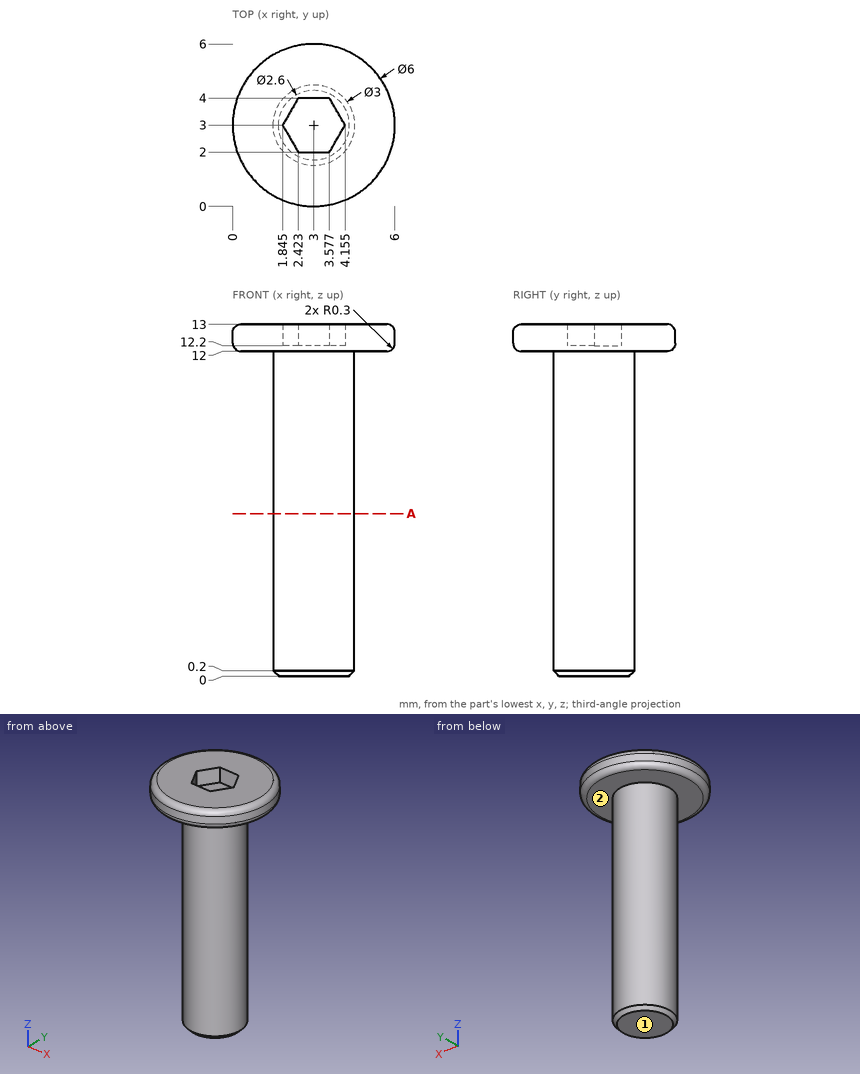
Study the drawing (mm; zero at the part's minimum x, y, z) and answer. A direction names the side the tool comes from. Give positions to 0.01 mm unless a question says otherwise; leave off trailing zeros. Write each loop counter-clockwise with the first axis right and the second up, starting at its lowest first coordinate (ties: lowest second). Pieces come first, ordered by that corner, then holes.
Item 1: Section A-A, the plane z = 6 is taken. Write down the section's boundary in (x, y).
Item 2: Find the intervals of material crossed by line 1 along Z through (x, y) = (3.75, 0.5); line 2 along X through (y, z) = (3.75, 12.5) (1 decimal); line 3 along Y through (x, z) = (3.5, 1) (1 decimal), in increasing order.
Item 3: Which of the six approach directions +Z, -Z, +X, -X, +Y, -Y give full straight-line access (tool end or side, diameter ignored) to the marked faces 1 and 2?
Item 4: Flat-ended cylindrical pins translate along their axes: P1, Ø1.5, axis at y = 3, z = 3, coming from the -X side; P2, Ø3, axis at y = 5, z = 3.5, coming from the -X side; P3, Ø3, axis at x = 3.5, z = 3, coming from the -Y side. Find the tip coordinate at first contact, or state that the pin passes through.
Completed:
1. outline: circle Ø3 at (3, 3)
2. line 1: z = 12 to 13
2. line 2: x = 0.1 to 2.3, 3.7 to 5.9
2. line 3: y = 1.6 to 4.4
3. face 1: -Z, +X, -X, +Y, -Y
3. face 2: -Z
4. P1: stops at x = 1.5
4. P2: stops at x = 1.59
4. P3: stops at y = 1.5
